The listing builds one solid part. Answer for the finished solid, in the listing's coordinates (mm). A direction names the side the tool comes from. Round coordinates to 2 decimals unless told otherwise and drop trailing zeros. Loops run counter-clockwise (first coordinate to the right, second up) from the corner with the lowest first, then second, coordinate; pieces in that order, holes last. Notation, with made-up numbers: M 48.25,83.5 L 87.25,83.5 A16 ccw 87.25,90.5 Z; hole C 81.5,-34.75 d6. An arc over 180 degrees is marked long. Answer as a JSON object with one key per item and string values.
```python
from build123d import *

# Parameters (mm, degrees)
BOSS_EXTRUDE1_DEPTH = 2.00000108
BOSS_EXTRUDE2_DEPTH = 2.00000108
BOSS_EXTRUDE3_DEPTH = 2.00000108
SKETCH4_R           = 1.499997
CUT_EXTRUDE1_DEPTH  = 9.070894964


with BuildPart() as part:
    # Sketch1 → Boss-Extrude1 (new body)
    with BuildSketch(Plane(origin=(0, 0, 0), x_dir=(1, 0, 0), z_dir=(0, 1, 0))):
        with BuildLine():
            Line((-3.61562396, -3.175), (3.61562396, -3.175))
            ThreePointArc((3.61562396, -3.175), (4.145954781, -2.955329781), (4.365625, -2.42499896))
            Line((4.365625, -2.42499896), (4.365625, 2.42499896))
            ThreePointArc((4.365625, 2.42499896), (4.145954781, 2.955329781), (3.61562396, 3.175))
            Line((3.61562396, 3.175), (-3.61562396, 3.175))
            ThreePointArc((-3.61562396, 3.175), (-4.145954781, 2.955329781), (-4.365625, 2.42499896))
            Line((-4.365625, 2.42499896), (-4.365625, -2.42499896))
            ThreePointArc((-4.365625, -2.42499896), (-4.145954781, -2.955329781), (-3.61562396, -3.175))
        make_face()
    extrude(amount=BOSS_EXTRUDE1_DEPTH)

    # Sketch2 → Boss-Extrude2 (add)
    with BuildSketch(Plane(origin=(0, 2.00000108, 0), x_dir=(1, 0, 0), z_dir=(0, 1, 0))):
        with BuildLine():
            Line((-1.50000081, 2.180197814), (-1.50000081, 2.17499946))
            Line((-1.50000081, 2.17499946), (1.50000081, 2.17499946))
            Line((1.50000081, 2.17499946), (1.50000081, 2.180197814))
            ThreePointArc((1.50000081, 2.180197814), (0, 2.79999948), (-1.50000081, 2.180197814))
        make_face()
        with BuildLine():
            Line((1.50000081, 2.17499946), (-1.50000081, 2.17499946))
            Line((-1.50000081, 2.17499946), (-1.50000081, 2.180197814))
            ThreePointArc((-1.50000081, 2.180197814), (-0.814899401, -1.287539785), (2.12499956, 0.67499992))
            ThreePointArc((2.12499956, 0.67499992), (1.962539705, 1.489899321), (1.50000081, 2.180197814))
            Line((1.50000081, 2.180197814), (1.50000081, 2.17499946))
        make_face()
        with BuildLine():
            Line((-1.50000081, 3.175), (-1.50000081, 2.180197814))
            ThreePointArc((-1.50000081, 2.180197814), (0, 2.79999948), (1.50000081, 2.180197814))
            Line((1.50000081, 2.180197814), (1.50000081, 3.175))
            Line((1.50000081, 3.175), (-1.50000081, 3.175))
        make_face()
    extrude(amount=BOSS_EXTRUDE2_DEPTH)

    # Sketch3 → Boss-Extrude3 (add)
    with BuildSketch(Plane(origin=(0, 4.00000216, 0), x_dir=(1, 0, 0), z_dir=(0, 1, 0))):
        with BuildLine():
            Line((-4.115624992, 2.42499896), (-4.115624992, -2.42499896))
            ThreePointArc((-4.115624992, -2.42499896), (-3.895954773, -2.955329781), (-3.365623952, -3.175))
            Line((-3.365623952, -3.175), (3.365623952, -3.175))
            ThreePointArc((3.365623952, -3.175), (3.895954773, -2.955329781), (4.115624992, -2.42499896))
            Line((4.115624992, -2.42499896), (4.115624992, 2.42499896))
            ThreePointArc((4.115624992, 2.42499896), (3.895954773, 2.955329781), (3.365623952, 3.175))
            Line((3.365623952, 3.175), (-3.365623952, 3.175))
            ThreePointArc((-3.365623952, 3.175), (-3.895954773, 2.955329781), (-4.115624992, 2.42499896))
        make_face()
    extrude(amount=BOSS_EXTRUDE3_DEPTH)

    # Sketch4 → Cut-Extrude1 (cut, through all)
    with BuildSketch(Plane.XZ):
        with Locations(Location((0, -0.67499992, 0), (0, 0, 270))):
            Circle(SKETCH4_R)
    extrude(amount=-CUT_EXTRUDE1_DEPTH, mode=Mode.SUBTRACT)


solid = part.part
```
Item 1: Which of the six approach directions +Z, -Z, +X, -X, +Y, -Y give full straight-line access (tool end or side, diameter ignored) to faces 5 (the face through (4.116, 5, 0)), 6 (the face through (-1.5, 3, -3)), 7 (the face through (4.366, 1, 0))?
Values follow:
{"face 5": "+Z, -Z, +X, +Y", "face 6": "-Z, -X", "face 7": "+Z, -Z, +X, +Y, -Y"}
Item 2: The part is cut by section A-A (x = 0). Give the vertices of the cut face in (y, z) (3 decimals).
Values follow:
{"outline": "M 0,-3.175 L 6,-3.175 L 6,-2.175 L 0,-2.175 Z; M 0,0.825 L 6,0.825 L 6,3.175 L 4,3.175 L 4,1.45 L 2,1.45 L 2,3.175 L 0,3.175 Z"}
Item 3: Flat-ended cylindrical pins translate along their axes: P1, Ø0.5, axis at y = 3.5, z = -2.5, coming from the -X side; P2, Ø1.6, axis at y = 5, z = 0, coming from the +X side; P3, Ø1.6, axis at y = 5, z = 0, coming from the -X side. Find the tip coordinate at first contact, or state that the pin passes through.
Values follow:
{"P1": "x = -1.5", "P2": "x = 4.12", "P3": "x = -4.12"}
Item 4: The part is cut by section D-D (z = 1.75). Give the vertices of the cut face in (x, y), then the cut area to 3 significant figures.
Values follow:
{"outline": "M -4.37,0 L 4.37,0 L 4.37,2 L -4.37,2 Z; M -4.12,4 L 4.12,4 L 4.12,6 L -4.12,6 Z", "area": "33.9 mm^2"}
Item 5: Straight lines are drawn through the part: line 1 (Y direction, x = 3.25, z = 0.75); line 2 (X direction, y = 2.25, z = -1.75); line 3 (X direction, y = 4.5, z = -1.25). For each, find the intervals that lie inside material, in ascending order.
Values follow:
{"line 1": "0 to 2, 4 to 6", "line 2": "-1.83 to -1.05, 1.05 to 1.83", "line 3": "-4.12 to -1.39, 1.39 to 4.12"}
Item 6: Determine the mould class of faces 1 (the face through (1.5, 3, -3)), 2 (the face through (-4.116, 5, 0)), 3 (the face through (0.451, 2.958, -2.106)), 4 (the face through (-1, 2, 1.4)) for opening direction X: released by +X, released by -X, zero draft, split by the parting line, or undercut.
Values follow:
{"face 1": "released by +X", "face 2": "released by -X", "face 3": "undercut", "face 4": "zero draft"}
Item 7: The part is cut by section C-C (z = 0.5). Give the vertices of the cut face in (x, y).
Values follow:
{"outline": "M -4.37,0 L -0.93,0 L -0.93,6 L -4.12,6 L -4.12,4 L -1.77,4 L -1.77,2 L -4.37,2 Z; M 0.93,0 L 4.37,0 L 4.37,2 L 1.77,2 L 1.77,4 L 4.12,4 L 4.12,6 L 0.93,6 Z"}
Item 8: The part is cut by section B-B (y = 4.75). Give the vertices of the cut face in (x, z) (3 decimals), then the cut area to 3 significant figures.
Values follow:
{"outline": "M -4.116,-2.425 A0.75 ccw -3.366,-3.175 L 3.366,-3.175 A0.75 ccw 4.116,-2.425 L 4.116,2.425 A0.75 ccw 3.366,3.175 L -3.366,3.175 A0.75 ccw -4.116,2.425 Z; hole C 0,-0.675 d3", "area": "44.7 mm^2"}
